from build123d import *

# Parameters (mm, degrees)
SKETCH1_W           = 190.5
SKETCH1_H           = 114.3
BOSS_EXTRUDE1_DEPTH = 31.75
SKETCH2_W           = 184.15
SKETCH2_H           = 107.95
CUT_EXTRUDE1_DEPTH  = 28.575
SKETCH3_R           = 5.08
BOSS_EXTRUDE2_DEPTH = 17.78
SKETCH4_R           = 3.175
CUT_EXTRUDE2_DEPTH  = 12.7
SKETCH5_W           = 19.05
SKETCH5_H           = 25.4
CUT_EXTRUDE3_DEPTH  = 12.7
SKETCH6_W           = 114.3
SKETCH6_H           = 54.61
BOSS_EXTRUDE3_DEPTH = 31.75
SKETCH7_W           = 107.95
SKETCH7_H           = 58.521622115
CUT_EXTRUDE4_DEPTH  = 28.575
SKETCH8_R           = 4.445
BOSS_EXTRUDE4_DEPTH = 21.971
SKETCH10_R          = 1.3716
CUT_EXTRUDE5_DEPTH  = 12.7
SKETCH11_R          = 4.604419826
BOSS_EXTRUDE5_DEPTH = 28.575
SKETCH12_R          = 2.064419826
CUT_EXTRUDE6_DEPTH  = 28.575


with BuildPart() as part:
    # Sketch1 → Boss-Extrude1 (new body)
    with BuildSketch(Plane(origin=(0, 0, 0), x_dir=(1, 0, 0), z_dir=(0, 1, 0))):
        with Locations((95.25, 57.15)):
            Rectangle(SKETCH1_W, SKETCH1_H)
    extrude(amount=BOSS_EXTRUDE1_DEPTH)

    # Sketch2 → Cut-Extrude1 (cut)
    with BuildSketch(Plane(origin=(0, 31.75, 0), x_dir=(1, 0, 0), z_dir=(0, 1, 0))):
        with Locations((95.25, 57.15)):
            Rectangle(SKETCH2_W, SKETCH2_H)
    extrude(amount=-CUT_EXTRUDE1_DEPTH, mode=Mode.SUBTRACT)

    # Sketch3 → Boss-Extrude2 (add)
    with BuildSketch(Plane(origin=(0, 3.175, 0), x_dir=(1, 0, 0), z_dir=(0, 1, 0))):
        with Locations((20.378923162, 94.615)):
            Circle(SKETCH3_R)
        with Locations((169.603923162, 94.615)):
            Circle(SKETCH3_R)
        with Locations((169.603923162, 19.685)):
            Circle(SKETCH3_R)
        with Locations((20.378923162, 19.685)):
            Circle(SKETCH3_R)
    extrude(amount=BOSS_EXTRUDE2_DEPTH)

    # Sketch4 → Cut-Extrude2 (cut)
    with BuildSketch(Plane(origin=(0, 20.955, 0), x_dir=(1, 0, 0), z_dir=(0, 1, 0))):
        with Locations((20.378923162, 94.615)):
            Circle(SKETCH4_R)
        with Locations((169.603923162, 94.615)):
            Circle(SKETCH4_R)
        with Locations((20.378923162, 19.685)):
            Circle(SKETCH4_R)
        with Locations((169.603923162, 19.685)):
            Circle(SKETCH4_R)
    extrude(amount=-CUT_EXTRUDE2_DEPTH, mode=Mode.SUBTRACT)

    # Sketch5 → Cut-Extrude3 (cut)
    with BuildSketch(Plane.XY):
        with Locations((64.135, 34.29)):
            Rectangle(SKETCH5_W, SKETCH5_H)
    extrude(amount=-CUT_EXTRUDE3_DEPTH, mode=Mode.SUBTRACT)

    # Sketch6 → Boss-Extrude3 (add)
    with BuildSketch(Plane.XZ):
        with Locations((133.35, -141.605)):
            Rectangle(SKETCH6_W, SKETCH6_H)
    extrude(amount=-BOSS_EXTRUDE3_DEPTH)

    # Sketch7 → Cut-Extrude4 (cut)
    with BuildSketch(Plane(origin=(0, 31.75, 0), x_dir=(1, 0, 0), z_dir=(0, 1, 0))):
        with Locations((133.35, 136.474188943)):
            Rectangle(SKETCH7_W, SKETCH7_H)
    extrude(amount=-CUT_EXTRUDE4_DEPTH, mode=Mode.SUBTRACT)

    # Sketch8 → Boss-Extrude4 (add)
    with BuildSketch(Plane(origin=(0, 3.175, 0), x_dir=(1, 0, 0), z_dir=(0, 1, 0))):
        with Locations((88.138, 127.0635)):
            Circle(SKETCH8_R)
        with Locations((163.068, 127.0635)):
            Circle(SKETCH8_R)
        with Locations((163.068, 158.242)):
            Circle(SKETCH8_R)
        with Locations((88.138, 158.242)):
            Circle(SKETCH8_R)
    extrude(amount=BOSS_EXTRUDE4_DEPTH)

    # Sketch10 → Cut-Extrude5 (cut)
    with BuildSketch(Plane(origin=(0, 25.146, 0), x_dir=(1, 0, 0), z_dir=(0, 1, 0))):
        with Locations((163.068, 127.0635)):
            Circle(SKETCH10_R)
        with Locations((88.138, 127.0635)):
            Circle(SKETCH10_R)
        with Locations((88.138, 158.242)):
            Circle(SKETCH10_R)
        with Locations((163.068, 158.242)):
            Circle(SKETCH10_R)
    extrude(amount=-CUT_EXTRUDE5_DEPTH, mode=Mode.SUBTRACT)

    # Sketch11 → Boss-Extrude5 (add)
    with BuildSketch(Plane(origin=(0, 3.175, 0), x_dir=(1, 0, 0), z_dir=(0, 1, 0))):
        with Locations((184.912, 5.588)):
            Circle(SKETCH11_R)
        with Locations((5.588, 5.588)):
            Circle(SKETCH11_R)
        with Locations((5.588, 108.712)):
            Circle(SKETCH11_R)
        with Locations((184.912, 163.322)):
            Circle(SKETCH11_R)
    extrude(amount=BOSS_EXTRUDE5_DEPTH)

    # Sketch12 → Cut-Extrude6 (cut)
    with BuildSketch(Plane(origin=(0, 31.75, 0), x_dir=(1, 0, 0), z_dir=(0, 1, 0))):
        with Locations((184.912, 5.588)):
            Circle(SKETCH12_R)
        with Locations((5.588, 5.588)):
            Circle(SKETCH12_R)
        with Locations((5.588, 108.712)):
            Circle(SKETCH12_R)
        with Locations((184.912, 163.322)):
            Circle(SKETCH12_R)
    extrude(amount=-CUT_EXTRUDE6_DEPTH, mode=Mode.SUBTRACT)


solid = part.part
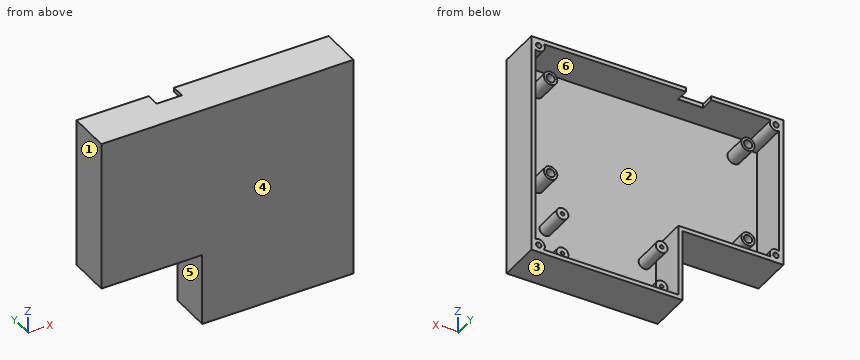
The model under review builds one solid part; all positions refer to its coordinate system, in mm. Face numbers are marked on the shaded views. A direction names the side the tool comes from. Give positions to 0.01 mm unless a question says otherwise; leave off trailing zeros. Order: outer loops, then holes, each group sorted by start corner. A loop starts at its lowest first (then second) coordinate and runs counter-clockwise, first axis right, second up. Notation, with made-up numbers: M -18.5,64 L 1.5,64 A23 cw 1.5,73 Z; hole C -11.5,83 d2. An arc over 180 degrees is marked long. Answer in a Markdown table with one row per item. Add a question column.
1. Add section A-A on x = 97. State the section outline as (y, z) points (3 decimals).
2. Machinability: for the marked faces 4, 5 and 6, which of the approach directions +Z, -Z, +X, -X, +Y, -Y give a long, thin tool a straight path to every point of the face, cutting with its end or side? Answer none if there is none.
3. Mouldability with a two-part tool opening along X and no side actions: class the marked faces 1, 2 and 3 as released by +X, released by -X, zero draft, split by the parting line, or undercut.
4. For pin 1 Ø10 at (x, z) = (162.5, -127.5) entering from +Y; pin 2 Ø5 at (x, z) = (22, -21) entering from +Y (3 decimals); pin 3 Ø5 at (x, z) = (20.38, -94.62) entering from +Y (3 decimals), all flat-tipped, find the tip position at first contact; note any pin that passes through.
5. To check wall thickness, follow line 1 along Z through (x, y) = (77.5, 17) (3 decimals); line 2 along Z through (x, y) = (112.5, 7) (3 decimals); line 3 along X through (y, z) = (11.5, -126.5) (3 decimals). State the ranges of each line that lie inside material, in increasing order.
6. Add section C-C on x = 170.5. State the section outline as (y, z) points (3 decimals), plus the area to 3 significant figures.
7. Add section B-B on z = -148. State the section outline as (x, y) points (3 decimals).
The answers:
| question | item | result |
|---|---|---|
| 1 | outline | M 0,-168.91 L 31.75,-168.91 L 31.75,-165.735 L 3.175,-165.735 L 3.175,-3.175 L 31.75,-3.175 L 31.75,0 L 0,0 Z |
| 2 | face 4 | +Z, -Z, +X, -X, -Y |
| 2 | face 5 | -Z, -X, +Y, -Y |
| 2 | face 6 | +Y |
| 3 | face 1 | released by -X |
| 3 | face 2 | undercut |
| 3 | face 3 | zero draft |
| 4 | pin 1 | y = 25.15 |
| 4 | pin 2 | y = 20.955 |
| 4 | pin 3 | y = 8.255 |
| 5 | line 1 | -168.91 to -111.125, -3.175 to 0 |
| 5 | line 2 | -168.91 to -165.735, -3.175 to 0 |
| 5 | line 3 | 76.2 to 79.375, 83.729 to 92.547, 158.659 to 167.477, 187.325 to 190.5 |
| 6 | outline | M 0,-168.91 L 31.75,-168.91 L 31.75,-165.735 L 3.175,-165.735 L 3.175,-99.615 L 20.955,-99.615 L 20.955,-97.661 L 8.255,-97.661 L 8.255,-91.569 L 20.955,-91.569 L 20.955,-89.615 L 3.175,-89.615 L 3.175,-24.685 L 20.955,-24.685 L 20.955,-22.731 L 8.255,-22.731 L 8.255,-16.639 L 20.955,-16.639 L 20.955,-14.685 L 3.175,-14.685 L 3.175,-3.175 L 31.75,-3.175 L 31.75,0 L 0,0 Z |
| 6 | area | 919 mm2 |
| 7 | outline | M 76.2,0 L 190.5,0 L 190.5,31.75 L 187.325,31.75 L 187.325,3.175 L 79.375,3.175 L 79.375,31.75 L 76.2,31.75 Z |
